Part model, mm, in its own coordinate system. Face numbers are marked on the shaded views. A direction names the side the tool comes from. Coordinates: 2 decimals unless noted, no trailing zeros. Order: outer loops, then holes, each group sorted by start corner. A loop starts at its lowest first (then second) coordinate and runs counter-clockwise, first axis right, second up.
1) Cut at A-A (y = 86). List the corners of the cut face in (x, z).
2) Pin check, flat tips, straight feed: pin 1 Ø22 at (x, y) = (2.5, 34.5) entering from +Z; pin 2 Ø1 at (x, y) = (-22.5, 9) entering from -Z; pin 3 Ø9 at (x, z) = (-5.5, -7) entering from +Y. Stop position of each tip, or through.
3) Mould opens along X. For the marked faces 1, 2 and 3 say: +X half, -X half, draft (parallel to the pull), parting line (faces both ways), or undercut.
4) Tool access for the marked faces 4, 5, 6, 7 and 8: list every direction of +Z, -Z, +X, -X, +Y, -Y with a clear straight run to the whole face (end or side of a thin tool).
5) Cut at B-B (x = -17). List the corners of the cut face in (y, z), and give its area (3 significant figures).
6) Cut at C-C (z = 0). List the corners of the cut face in (x, y).
7) Cut at D-D (y = 51.5). List the corners of the cut face in (x, z), and give its area (3 significant figures).
8) Wall check: L1, parallel to Z at x = -2, y = 69; L2, parallel to Y at x = 6.5, z = 12.75. Give the ranges that are in metal, low to high.
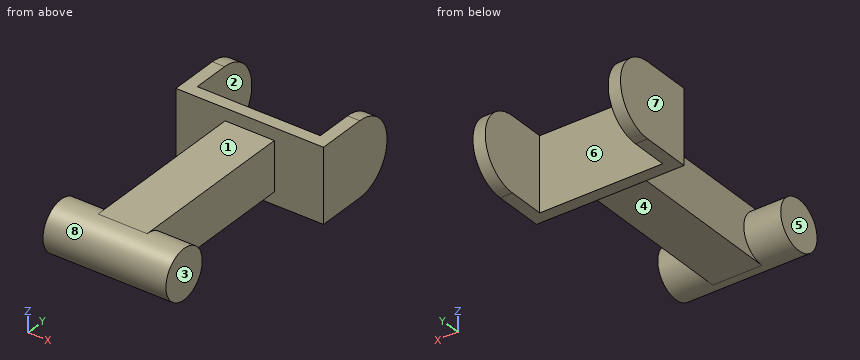
Autodesk Inventor part; units mm, degrees
ref_plane "YZ Plane" through (0, 0, 0) normal (1, 0, 0) x (0, 1, 0)
ref_plane "XZ Plane" through (0, 0, 0) normal (0, 1, 0) x (-1, 0, 0)
ref_plane "XY Plane" through (0, 0, 0) normal (0, 0, 1) x (1, 0, 0)
sketch "스케치7" plane through (0, 0, 0) normal (1, 0, 0) x (0, 1, 0)
  circle A0 centre (0, 0) radius 10
  dimension "d29" = 20
extrude "돌출7" add sketch "스케치7" along normal mid plane 50
sketch "스케치8" plane through (0, 0, 0) normal (0, 1, 0) x (-1, 0, 0)
  line L0 (25, 10) -> (-25, 10)
  line L1 (25, -10) -> (-25, -10)
  line L2 (10, 10) -> (-10, 10)
  line L3 (-10, 10) -> (-10, -10)
  line L4 (-10, -10) -> (10, -10)
  line L5 (10, -10) -> (10, 10)
  line L6 (25, -10) -> (25, 10)
  point P0 (0, 0)
  dimension "d32" = 20
  dimension "d33" = 15
extrude "돌출8" add sketch "스케치8" along normal blind 70 contours L5 L1 L3 L0
sketch "스케치9" plane through (0, 70, 0) normal (0, 1, 0) x (1, 0, 0)
  line L0 (-30, -15) -> (30, -15)
  line L1 (30, -15) -> (30, 15)
  line L2 (30, 15) -> (-30, 15)
  line L3 (-30, 15) -> (-30, -15)
  line L4 (-30, -15) -> (30, 15) construction
  line L5 (30, -15) -> (-30, 15) construction
  point P0 (0, 0)
  dimension "d36" = 60
  dimension "d37" = 30
extrude "돌출9" add sketch "스케치9" along normal blind 5
sketch "스케치10" plane through (-30, 70, -15) normal (-1, 0, 0) x (0, 0, 1)
  line L0 (0, 5) -> (30, 5)
  line L1 (30, 5) -> (30, 20)
  line L2 (30, 20) -> (0, 20)
  line L3 (0, 20) -> (0, 5)
  arc A0 (30, 20) -> (0, 20) centre (15, 20) ccw
  point P0 (15, -70)
  dimension "d40" = 30
  dimension "d41" = 15
extrude "돌출10" add sketch "스케치10" against normal blind 5
mirror "미러3" about plane through (0, 0, 0) normal (1, 0, 0) of "돌출10"
properties part number "L2_0.1" material "ABS 플라스틱"
Geometry check:
1. outline: (-30, -15) - (-25, -15) - (-25, 15) - (-30, 15) - close; (25, -15) - (30, -15) - (30, 15) - (25, 15) - close
2. pin 1: stops at z = 10
2. pin 2: stops at z = -5.27
2. pin 3: stops at y = 75
3. face 1: draft
3. face 2: undercut
3. face 3: +X half
4. face 4: -Z, +X, -X, -Y
4. face 5: +Z, -Z, -X, -Y
4. face 6: +Z, -Z, +Y
4. face 7: +Z, -Z, -X, +Y, -Y
4. face 8: none
5. outline: circle Ø20 at (0, 0); (70, -15) - (75, -15) - (75, 15) - (70, 15) - close
5. area: 464 mm2
6. outline: (-30, 70) - (-10, 70) - (-10, 10) - (-25, 10) - (-25, -10) - (25, -10) - (25, 10) - (10, 10) - (10, 70) - (30, 70) - (30, 105) - (25, 105) - (25, 75) - (-25, 75) - (-25, 105) - (-30, 105) - close
7. outline: (-10, -10) - (10, -10) - (10, 10) - (-10, 10) - close
7. area: 400 mm2
8. L1: z = -10 to 10
8. L2: y = 70 to 75
